Source: CAD feature listing. Evaluate the final solid. Frame: model axes, mm. A direction names the side the tool comes from. Round coordinates to 2 decimals unless told otherwise and drop trailing zeros. Order: outer loops, then holes, each group sorted by start corner. A loop starts at its lowest first (then second) coordinate and runs counter-clockwise, first axis right, second up. Notation, with made-up numbers: M 72,-8.5 L 99,-8.5 A29 cw 99,21.5 Z; hole C -26.5,-6 d10. An arc over 180 degrees is marked long. Use CSV: the item, a comma, the result in double quotes. Start each with the question number.
```python
from build123d import *

# Parameters (mm, degrees)
SKETCH1_R           = 2
BOSS_EXTRUDE1_DEPTH = 13
SKETCH2_R           = 47.5
CUT_EXTRUDE1_DEPTH  = 10
SKETCH3_R           = 42.5
CUT_EXTRUDE2_DEPTH  = 10


with BuildPart() as part:
    # Sketch1 → Boss-Extrude1 (new body)
    # profile 1 of 4: a face of its own
    with BuildSketch(Plane(origin=(0, 0, 0), x_dir=(1, 0, 0), z_dir=(0, 1, 0))):
        with BuildLine():
            ThreePointArc((61.367242208, -6.544599037), (65.988588721, 0.043478359), (61.35856476, 6.625460242))
            ThreePointArc((61.35856476, 6.625460242), (55.933608349, 10.171878458), (52.687221143, 15.781531238))
            ThreePointArc((52.687221143, 15.781531238), (-54.999988062, -0.036238224), (52.707971563, -15.712088776))
            ThreePointArc((52.707971563, -15.712088776), (55.946963812, -10.098162928), (61.367242208, -6.544599037))
        make_face()
        with Locations(Location((58.98859024, 0.038866222, 0), (0, 0, 270))):
            Circle(SKETCH1_R, mode=Mode.SUBTRACT)
    # profile 2 of 4: a face of its own
    with BuildSketch(Plane(origin=(0, 0, 0), x_dir=(1, 0, 0), z_dir=(0, 1, 0))):
        with BuildLine():
            ThreePointArc((6.625460242, -61.35856476), (10.171878458, -55.933608349), (15.781531238, -52.687221143))
            ThreePointArc((15.781531238, -52.687221143), (0.036238224, -54.999988062), (-15.712088776, -52.707971563))
            ThreePointArc((-15.712088776, -52.707971563), (-10.098162928, -55.946963812), (-6.544599037, -61.367242208))
            ThreePointArc((-6.544599037, -61.367242208), (0.043478359, -65.988588721), (6.625460242, -61.35856476))
        make_face()
        with Locations(Location((0.038866222, -58.98859024, 0), (0, 0, 270))):
            Circle(SKETCH1_R, mode=Mode.SUBTRACT)
    # profile 3 of 4: a face of its own
    with BuildSketch(Plane(origin=(0, 0, 0), x_dir=(1, 0, 0), z_dir=(0, 1, 0))):
        with BuildLine():
            ThreePointArc((-52.687221143, -15.781531238), (-54.999988062, -0.036238224), (-52.707971563, 15.712088776))
            ThreePointArc((-52.707971563, 15.712088776), (-55.946963812, 10.098162928), (-61.367242208, 6.544599037))
            ThreePointArc((-61.367242208, 6.544599037), (-65.988588721, -0.043478359), (-61.35856476, -6.625460242))
            ThreePointArc((-61.35856476, -6.625460242), (-55.933608349, -10.171878458), (-52.687221143, -15.781531238))
        make_face()
        with Locations(Location((-58.98859024, -0.038866222, 0), (0, 0, 270))):
            Circle(SKETCH1_R, mode=Mode.SUBTRACT)
    # profile 4 of 4: a face of its own
    with BuildSketch(Plane(origin=(0, 0, 0), x_dir=(1, 0, 0), z_dir=(0, 1, 0))):
        with BuildLine():
            ThreePointArc((-15.781531238, 52.687221143), (-0.036238224, 54.999988062), (15.712088776, 52.707971563))
            ThreePointArc((15.712088776, 52.707971563), (10.098162928, 55.946963812), (6.544599037, 61.367242208))
            ThreePointArc((6.544599037, 61.367242208), (-0.043478359, 65.988588721), (-6.625460242, 61.35856476))
            ThreePointArc((-6.625460242, 61.35856476), (-10.171878458, 55.933608349), (-15.781531238, 52.687221143))
        make_face()
        with Locations(Location((-0.038866222, 58.98859024, 0), (0, 0, 270))):
            Circle(SKETCH1_R, mode=Mode.SUBTRACT)
    extrude(amount=-BOSS_EXTRUDE1_DEPTH)

    # Sketch2 → Cut-Extrude1 (cut)
    with BuildSketch(Plane(origin=(0, 0, 0), x_dir=(1, 0, 0), z_dir=(0, 1, 0))):
        with Locations(Location((0, 0, 0), (0, 0, 270))):
            Circle(SKETCH2_R)
    extrude(amount=-CUT_EXTRUDE1_DEPTH, mode=Mode.SUBTRACT)

    # Sketch3 → Cut-Extrude2 (cut)
    with BuildSketch(Plane(origin=(0, -10, 0), x_dir=(1, 0, 0), z_dir=(0, 1, 0))):
        with Locations(Location((0, 0, 0), (0, 0, 270))):
            Circle(SKETCH3_R)
    extrude(amount=-CUT_EXTRUDE2_DEPTH, mode=Mode.SUBTRACT)


solid = part.part
```
(1) Section D-D on z = 45. Return loops of the section in (x, y), plus the area to 3 significant figures.
(2) Reachability of faces 5 (the face through (-46.37, -4.93, -10.3)), 6 (the face through (-10.1, -6.4, -56)) from +Z, -Z, +X, -X, +Y, -Y: full face, straight path, thin tool, end or side. Return the list, or none.
(3) Line query: line 1 along X through (y, z) = (-11.5, 0); line 2 along X through (y, z) = (-2.5, 0); line 3 along Y through (x, z) = (13, -43.5). Output: solid intervals per line, ascending.
(4) Section B-B on x = 11.5. Return loops of the section in (y, z), plus the area to 3 significant figures.
(5) Section C-C on y = -6.25. Return loops of the section in (x, z), plus the area to 3 significant figures.
(6) Contact query for flat-ended pins moving along their axis: P1, Ø4.5, axis at x = 0.04, z = 58.99, coming from the -Y side; P2, Ø4, axis at x = 52.5, y = -8, coming from the +Z side; P3, Ø6, axis at y = -10, z = -19, coming from the +X side; P4, Ø6, axis at x = 20.5, y = -10.5, coming from the -Z side. Output: stop coordinate, or through.
(7) Draft query along X for faces 1 (the face through (38.65, -6.41, 39.13)), 2 (the face through (-24.4, -10, -35.4)), 3 (the face through (60.97, -6.41, -0.3)), 4 (the face through (19, 0, 44)). Return one class per face: pulls with the +X half, pulls with the -X half, needs draft (parallel to the pull), parting line crosses it, or undercut.
(8) Section A-A on z = 13. Return loops of the section in (x, y), plus the area to 3 significant figures.
Results below:
1,outline,"M -31.62,-13 L 31.62,-13 L 31.62,0 L 15.21,0 L 15.21,-10 L -15.21,-10 L -15.21,0 L -31.62,0 Z"
1,area,"518 mm2"
2,face 5,"+Y"
2,face 6,"-Z, -X, +Y, -Y"
3,line 1,"x = -65.99 to -60.99, -56.99 to -42.5, 42.5 to 56.99, 60.99 to 65.99"
3,line 2,"x = -65.99 to -60.99, -56.99 to -47.5, 47.5 to 56.99, 60.99 to 65.99"
3,line 3,"y = -13 to -10"
4,outline,"M -13,-54.79 L 0,-54.79 L 0,-46.09 L -10,-46.09 L -10,-40.91 L -13,-40.91 Z; M -13,40.91 L -10,40.91 L -10,46.09 L 0,46.09 L 0,54.82 L -13,54.82 Z"
4,area,"258 mm2"
5,outline,"M -61.37,-6.54 A14 cw -52.71,-15.71 A55 ccw -15.78,-52.69 A14 cw -6.63,-61.36 A7 ccw 6.54,-61.37 A14 cw 15.71,-52.71 A55 ccw 52.69,-15.78 A14 cw 61.36,-6.63 A7 ccw 61.37,6.54 A14 cw 52.71,15.71 A55 ccw 15.78,52.69 A14 cw 6.63,61.36 A7 ccw -6.54,61.37 A14 cw -15.71,52.71 A55 ccw -52.69,15.78 A14 cw -61.36,6.63 A7 ccw Z; hole C -58.99,0.04 d4; hole C 0,0 d95; hole C -0.04,-58.99 d4; hole C 0.04,58.99 d4; hole C 58.99,-0.04 d4"
5,area,"3,020 mm2"
6,P1,"stops at y = -13"
6,P2,"stops at z = 21.79"
6,P3,"stops at x = 52.62"
6,P4,"stops at z = -52.14"
7,face 1,"pulls with the +X half"
7,face 2,"undercut"
7,face 3,"undercut"
7,face 4,"needs draft"
8,outline,"M -53.86,-13 L -40.46,-13 L -40.46,-10 L -45.69,-10 L -45.69,0 L -53.86,0 Z; M 40.46,-13 L 53.84,-13 L 53.84,0 L 45.69,0 L 45.69,-10 L 40.46,-10 Z"
8,area,"244 mm2"
